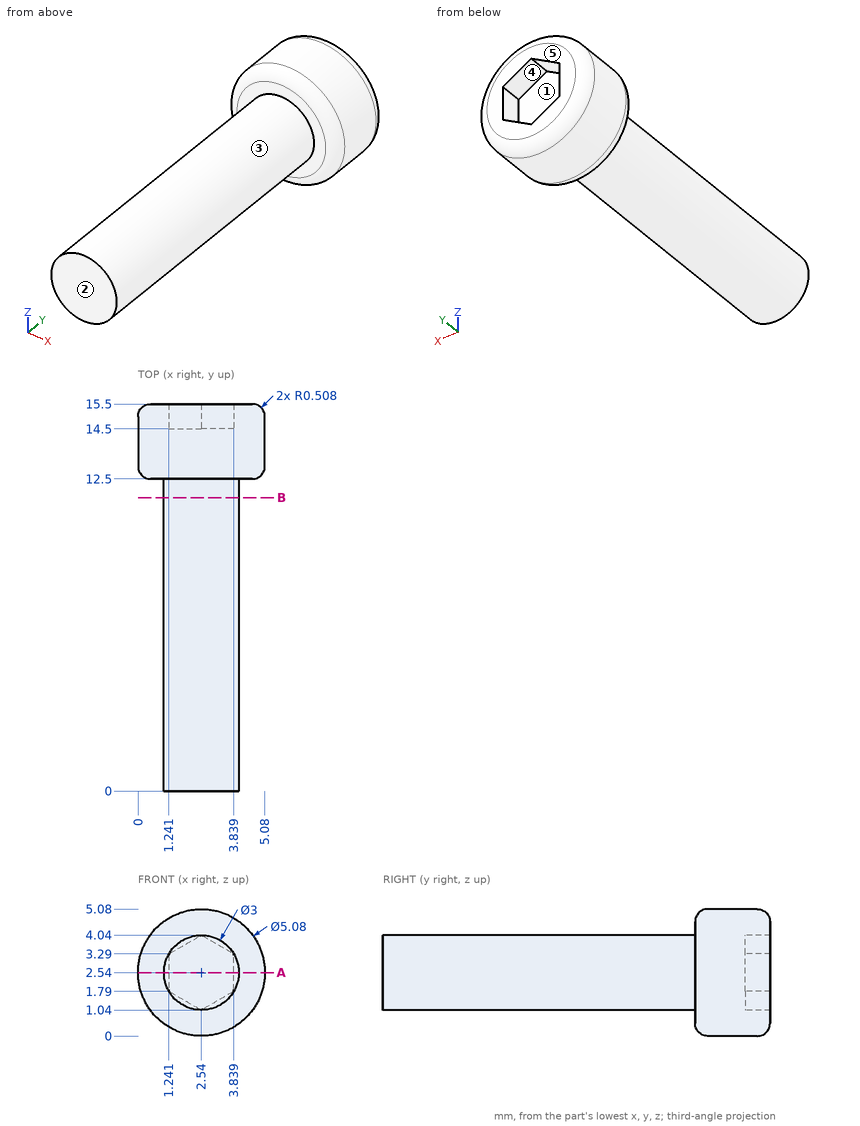
Drawing for the job (mm, zero at the part's lowest x, y, z). A direction names the side the tool comes from. Give positions to 0.01 mm unless a question says otherwise; leave off trailing zeros. Loops run counter-clockwise (first coordinate to the right, second up) from the corner with the lowest first, then second, coordinate; pieces in that order, holes last.
1) Drop flat-ended pins along their axis: P1, Ø3, axis at x = 1.5, y = 6, coming from the -Z side; P2, Ø2, axis at x = 2, y = 8.5, coming from the +Z side; P3, Ø1.5, axis at y = 10.5, z = 3.5, coming from the +X side (1 decimal). Give the stop position or say it passes through.
Values follow:
P1: stops at z = 1.04
P2: stops at z = 4.04
P3: stops at x = 4
2) Band-saw the part on B-B on y = 11.75. List the corners of the cut face in (x, z).
Values follow:
outline: circle Ø3 at (2.54, 2.54)
3) 3-axis set-ups, long thin cutter, end or side, ignore diameter. For the marked faces 1 and 2: which of +Z, -Z, +X, -X, +Y, -Y reach the whole face in a straight line?
Values follow:
face 1: +Y
face 2: +Z, -Z, +X, -X, -Y
4) Probe line 1 along Y through (x, z) = (3.1, 0.7); line 2 along Y through (x, z) = (2.35, 3.4); line 3 along X through (y, z) = (0.5, 2.65). List the from-to ranges inside material, lowest first.
Values follow:
line 1: y = 12.5 to 15.5
line 2: y = 0 to 14.5
line 3: x = 1.04 to 4.04
5) Two-plate mould, pull along X, no slides. Class the marked faces 3, 4 and 5: released by +X, released by -X, zero draft, split by the parting line, or undercut.
Values follow:
face 3: split by the parting line
face 4: undercut
face 5: zero draft
6) Band-saw the part on A-A on z = 2.54. List the corners of the cut face in (x, y).
Values follow:
outline: (0, 13.01) arc R0.51 ccw to (0.51, 12.5) - (1.04, 12.5) - (1.04, 0) - (4.04, 0) - (4.04, 12.5) - (4.57, 12.5) arc R0.51 ccw to (5.08, 13.01) - (5.08, 14.99) arc R0.51 ccw to (4.57, 15.5) - (3.84, 15.5) - (3.84, 14.5) - (1.24, 14.5) - (1.24, 15.5) - (0.51, 15.5) arc R0.51 ccw to (0, 14.99) - close
